Autodesk Inventor part; units mm, degrees
ref_plane "YZ Plane" through (0, 0, 0) normal (1, 0, 0) x (0, 1, 0)
ref_plane "XZ Plane" through (0, 0, 0) normal (0, 1, 0) x (-1, 0, 0)
ref_plane "XY Plane" through (0, 0, 0) normal (0, 0, 1) x (1, 0, 0)
sketch "Sketch3" plane through (0, 0, 0) normal (0, 0, 1) x (1, 0, 0)
  line L0 (0, 0) -> (33.6, 0)
  line L1 (33.6, 0) -> (33.6, 58.6)
  line L2 (33.6, 58.6) -> (0, 58.6)
  line L3 (0, 58.6) -> (0, 0)
  line L4 (-2, 60.6) -> (35.6, 60.6)
  line L5 (35.6, 60.6) -> (35.6, -2)
  line L6 (35.6, -2) -> (-2, -2)
  line L7 (-2, -2) -> (-2, 60.6)
  dimension "d36" = 33.6
  dimension "d37" = 58.6
  dimension "d38" = 2
extrude "Extrusion3" add sketch "Sketch3" along normal blind 46
sketch "Sketch4" plane through (0, 0, 0) normal (0, 0, -1) x (-1, 0, 0)
  circle A0 centre (-16.775, 44.825) radius 13.5
  line L0 (0, 58.6) -> (-33.6, 58.6)
  line L1 (0, 0) -> (0, 58.6)
  line L2 (-33.6, 58.6) -> (-33.6, 0)
  line L3 (-33.6, 6.5) -> (0, 6.5)
  line L4 (0, 0) -> (0, 58.6)
  line L5 (-33.6, 0) -> (0, 0)
  line L6 (-33.6, 0) -> (0, 0)
  line L7 (-33.6, 6.5) -> (0, 6.5)
  line L8 (0, 6.5) -> (0, 0)
  line L9 (0, 0) -> (-33.6, 0)
  line L10 (-33.6, 0) -> (-33.6, 6.5)
  line L11 (-35.6, 60.6) -> (2, 60.6)
  line L12 (2, 60.6) -> (2, -2)
  line L13 (-35.6, 60.6) -> (2, 60.6)
  line L14 (2, 60.6) -> (2, -2)
  line L15 (2, -2) -> (-35.6, -2)
  line L16 (-35.6, -2) -> (-35.6, 60.6)
  line L17 (-33.6, 58.6) -> (-33.6, 0)
  line L18 (-33.6, 0) -> (-33.6, -2)
  line L19 (0, 0) -> (0, -2)
  line L20 (2, -2) -> (-35.6, -2)
  point P0 (0, 6.5)
  dimension "d41" = 27
  dimension "d42" = 13.775
  dimension "d43" = 16.775
  dimension "d44" = 6.5
extrude "Extrusion4" add sketch "Sketch4" along normal blind 2 contours L1 L3 L2 L0 | L0 L2 L18 L15 L16 L11 L12 L19 L1
sketch "Sketch5" plane through (-2, 60.6, 46) normal (0, 1, 0) x (1, 0, 0)
  line L0 (0, 0) -> (37.6, 0)
  line L1 (37.6, 48) -> (37.6, 0)
  line L2 (0, 0) -> (37.6, 0)
  line L3 (37.6, 0) -> (37.6, 48)
  line L4 (37.6, 48) -> (0, 48)
  line L5 (0, 48) -> (0, 0)
  point P0 (2, 46)
extrude "Extrusion5" add sketch "Sketch5" along normal blind 0.5
sketch "Sketch6" plane through (0, 0, 46) normal (0, 0, 1) x (1, 0, 0)
  line L0 (-2, -2) -> (35.6, -2)
  line L1 (35.6, -2) -> (35.6, 6.3)
  line L2 (35.6, 6.3) -> (-2, 6.3)
  line L3 (-2, 6.3) -> (-2, -2)
  line L4 (0, 6.5) -> (0, -2)
  line L5 (0, 6.3) -> (0, -2)
  line L6 (35.6, -2) -> (33.6, -2)
  line L7 (33.6, 6.3) -> (33.6, -2)
  point P0 (0, 0)
  dimension "d56" = 8.3
extrude "Extrusion6" cut sketch "Sketch6" against normal blind 2.1 contours L4 L2 L7 L0
sketch "Sketch7" plane through (-2, -2, -2) normal (-1, 0, 0) x (0, 0, 1)
  line L0 (0, 37.3) -> (6, 37.3)
  line L1 (0, 24.3) -> (6, 24.3)
  line L2 (6, 37.3) -> (6, 24.3)
  line L3 (2, 33.325) -> (2, 60.325)
  line L4 (48, 0) -> (0, 0)
  line L5 (2, 37.3) -> (2, 24.3)
  line L6 (0, 37.3) -> (0, 24.3)
  line L7 (0, 33.325) -> (0, 60.325)
  point P0 (2, 2)
  point P1 (3, 24.3)
  point P2 (2, 37.3)
  dimension "d59" = 6
  dimension "d60" = 13
  dimension "d61" = 24.3
extrude "Extrusion7" cut sketch "Sketch7" against normal up to surface (2 mm away) contours L0 L2 L1 L5 L3
fillet "Fillet3" radius 2 1 edges at (35.6, 61.1, 22)
fillet "Fillet4" radius 2 1 edges at (-2, 61.1, 22)
properties part number "Base_Demo_1"
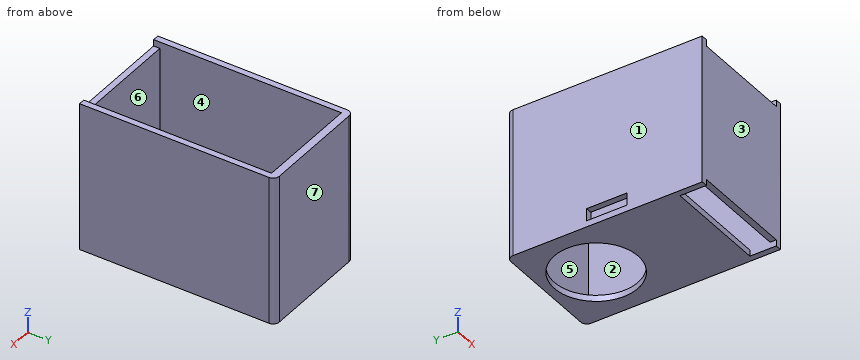
Here's how the part is built. I have some questions about the finished solid (model axes, mm). Face numbers are marked on the shaded views. A direction names the side the tool comes from. Coordinates: 2 decimals unless noted, no trailing zeros. Order: outer loops, then holes, each group sorted by start corner. A loop starts at its lowest first (then second) coordinate and runs counter-clockwise, first axis right, second up. Notation, with made-up numbers: M 47.25,64.25 L 98.25,64.25 A22 cw 98.25,100.25 Z; hole C 13,88 d8. An arc over 180 degrees is marked long. Answer as a JSON object with one key per item and string values. Group by question number.
(1) Suppose I cut it at D-D, the plane y = 13. Please give me the cut outline in (x, z).
(2) Suppose I cut it at A-A, the plane y = 23.5. Please give me the cut outline in (x, z), then the cut area to 3 significant figures.
(3) If we mould it in two halves opening along Y, with no side actions, what happens to the marked faces 1, 2, 3 and 4? For each: released by +Y, released by -Y, zero draft, split by the parting line, or undercut.
(4) Suppose I cut it at B-B, the plane x = 27.5. Please give me the cut outline in (y, z).
(5) I need wall thicknesses on probe 1 along X at (y, z) = (22, 2.5); probe 2 along Y at (x, z) = (20.5, 41.5); probe 3 along Z at (x, y) = (13.5, 25.5). Which ranges of each line are inside material? Lowest first, please.
(6) For pin 1 (1.6 mm diameter, centred on x = 19, z = -1, fed in from -Y); pin 2 (0.6 mm diameter, centred on x = 14, y = -1, fed in from +Z); pin 3 (12 mm diameter, centred on x = 8.5, y = 48.5, fed in from +Z), each with a flat end and sliding along its axis, tell me the tip position at first contact or that it passes through.
(7) Which directions (+Z, -Z, +X, -X, +Y, -Y) give clear straight access to the entire face, cutting with the end or side of a thin tool? Please do the marked faces 5, 6 and 7.
(8) Suppose I cut it at C-C, the plane z = 18.5. Please give me the cut outline in (x, y), then the cut area to 3 significant figures.
Values found:
{
 "1": {"outline": "M -2,-2 L 35.6,-2 L 35.6,46 L 33.6,46 L 33.6,0 L 0,0 L 0,46 L -2,46 Z"},
 "2": {"outline": "M -2,-2 L 35.6,-2 L 35.6,46 L 33.6,46 L 33.6,0 L -2,0 Z; M -2,4 L 0,4 L 0,46 L -2,46 Z", "area": "251 mm^2"},
 "3": {"face 1": "zero draft", "face 2": "undercut", "face 3": "released by -Y", "face 4": "undercut"},
 "4": {"outline": "M -2,0 L 0,0 L 0,43.9 L -2,43.9 Z; M 6.5,-2 L 36.63,-2 L 36.63,0 L 6.5,0 Z; M 53.02,-2 L 61.1,-2 L 61.1,46 L 58.6,46 L 58.6,0 L 53.02,0 Z"},
 "5": {"probe 1": "x = -2 to 0, 33.6 to 35.6", "probe 2": "y = -2 to 0, 58.6 to 61.1", "probe 3": "z = -2 to 0"},
 "6": {"pin 1": "stops at y = 6.5", "pin 2": "stops at z = 43.9", "pin 3": "stops at z = 0"},
 "7": {"face 5": "+Z", "face 6": "+Z, -Z", "face 7": "+Z, -Z, +X, -X, +Y"},
 "8": {"outline": "M -2,-2 L 35.6,-2 L 35.6,59.1 A2 ccw 33.6,61.1 L 0,61.1 A2 ccw -2,59.1 Z; hole M 0,0 L 33.6,0 L 33.6,58.6 L 0,58.6 Z", "area": "402 mm^2"}
}
